Geometry check sheet. Reference: drawing and pictorial views, mm from the part's lowest x, y, z. Round coordinates to 2 decimals unless told otherwise and drop trailing zeros. Write each loop counter-clockwise with the first axis right and the second up, starting at its lowest first coordinate (ties: lowest second). Pieces come first, ordered by that corner, then holes. Notation, with made-up numbers: M 6.5,-31.5 L 41.5,-31.5 A11 cw 41.5,-19.5 Z; hole C 66.25,4 d8. An arc over 180 degrees is marked long. Answer in a Markdown table with one row per item.
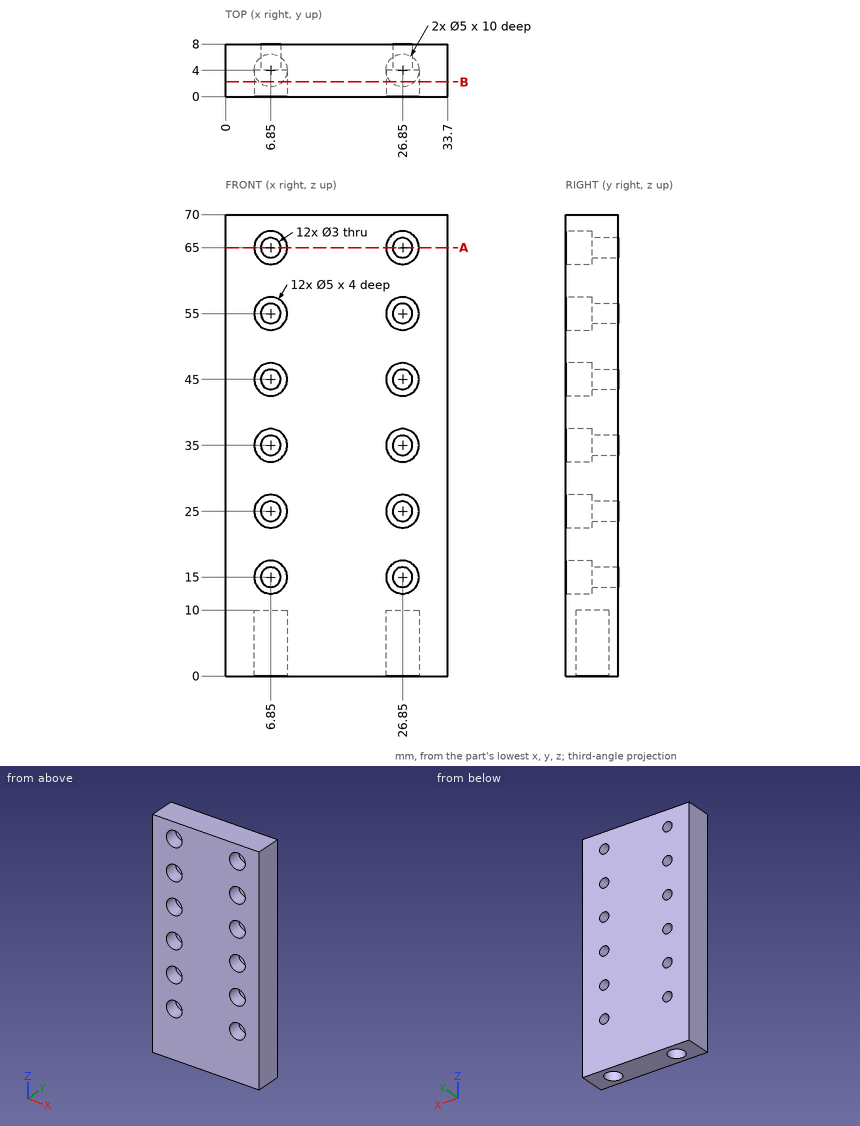
1. Section check A-A, the plane z = 65. Record the cut outline in (x, y).
Found:
| item | result |
|---|---|
| outline | M 0,0 L 4.35,0 L 4.35,4 L 5.35,4 L 5.35,8 L 0,8 Z; M 8.35,4 L 9.35,4 L 9.35,0 L 24.35,0 L 24.35,4 L 25.35,4 L 25.35,8 L 8.35,8 Z; M 28.35,4 L 29.35,4 L 29.35,0 L 33.7,0 L 33.7,8 L 28.35,8 Z |
2. Go/stop test with a flat-tipped pin: pin 1 (4 mm diameter, centred on x = 7, z = 55, fed in from -Y). Record where the tip stops, or that it passes through.
Found:
| item | result |
|---|---|
| pin 1 | stops at y = 4 |
3. Scan lines: L1, parallel to X at y = 2.3, z = 45; L2, parallel to X at y = 1.5, z = 63; L3, parallel to Y at x = 4.5, z = 55. Record each from-to range of solid material in increasing order.
Found:
| item | result |
|---|---|
| L1 | x = 0 to 4.35, 9.35 to 24.35, 29.35 to 33.7 |
| L2 | x = 0 to 5.35, 8.35 to 25.35, 28.35 to 33.7 |
| L3 | y = 4 to 8 |
4. Section check B-B, the plane y = 2.25. Count the separate pieces of the cut face and the enclosed holes in it, and give its area (3 significant figures).
Found:
| item | result |
|---|---|
| separate pieces | 1 |
| enclosed holes | 12 |
| area | 2,050 mm2 |
